```python
from build123d import *

# Parameters (mm, degrees)
ESQUISSE2_W        = 11.89
ESQUISSE2_H        = 4.55
BOSS_EXTRU_1_DEPTH = 1.5
ESQUISSE7_W        = 7.59
ESQUISSE7_H        = 3.5
BOSS_EXTRU_2_DEPTH = 1
ESQUISSE8_W        = 0.56222282
ESQUISSE8_H        = 1.99
BOSS_EXTRU_4_DEPTH = 7.3
CONG_6_R           = 0.995
ESQUISSE12_R       = 0.44
BOSS_EXTRU_5_DEPTH = 1.21


with BuildPart() as part:
    # Esquisse2 → Boss.-Extru.1 (new body)
    with BuildSketch(Plane(origin=(0, 0, 0), x_dir=(0, 0, -1), z_dir=(1, 0, 0))):
        with Locations((-5.945, 2.275)):
            Rectangle(ESQUISSE2_W, ESQUISSE2_H)
    extrude(amount=BOSS_EXTRU_1_DEPTH)

    # Esquisse7 → Boss.-Extru.2 (add)
    with BuildSketch(Plane(origin=(1.5, 0, 0), x_dir=(0, 0, -1), z_dir=(1, 0, 0))):
        with Locations((-5.945, 2.275)):
            Rectangle(ESQUISSE7_W, ESQUISSE7_H)
    extrude(amount=BOSS_EXTRU_2_DEPTH)

    # Esquisse8 → Boss.-Extru.4 (add)
    with BuildSketch(Plane(origin=(5.3, 0, 0), x_dir=(0, 0, -1), z_dir=(1, 0, 0))):
        with Locations((-6.93462953, 2.275)):
            Rectangle(ESQUISSE8_W, ESQUISSE8_H)
        with Locations((-2.97611141, 2.275)):
            Rectangle(ESQUISSE8_W, ESQUISSE8_H)
        with Locations((-8.91388859, 2.275)):
            Rectangle(ESQUISSE8_W, ESQUISSE8_H)
        with Locations((-4.95537047, 2.275)):
            Rectangle(ESQUISSE8_W, ESQUISSE8_H)
    extrude(amount=-BOSS_EXTRU_4_DEPTH)

    # Congé6
    cong_6_edges = [part.edges().sort_by_distance(p)[0] for p in [
        (5.3, 1.28, 2.97611141),
        (5.3, 1.28, 4.95537047),
        (5.3, 1.28, 6.93462953),
        (5.3, 1.28, 8.91388859),
        (5.3, 3.27, 8.91388859),
        (5.3, 3.27, 6.93462953),
        (5.3, 3.27, 4.95537047),
        (5.3, 3.27, 2.97611141),
    ]]
    fillet(cong_6_edges, radius=CONG_6_R - 0.0001)  # a hair under: the kernel refuses the full size

    # Esquisse12 → Boss.-Extru.5 (add)
    with BuildSketch(Plane.ZY):
        with Locations(Location((2.135, 4.06, 0), (0, 0, 180))):
            Circle(ESQUISSE12_R)
        with Locations(Location((9.755, 0.49, 0), (0, 0, 180))):
            Circle(ESQUISSE12_R)
    extrude(amount=BOSS_EXTRU_5_DEPTH)


solid = part.part
```
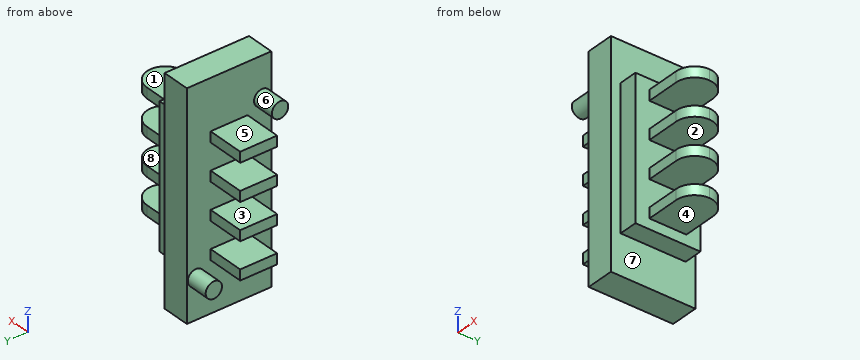
Design review of the part built by this model. Coordinates are the model's own, in mm. Face numbers are marked on the shaded views. A direction names the side the tool comes from. Give positions to 0.01 mm unless a question says otherwise; leave off trailing zeros. Order: outer loops, then holes, each group sorted by start corner. A loop starts at its lowest first (then second) coordinate and runs counter-clockwise, first axis right, second up. Notation, with made-up numbers: (5, 67.25) - (9, 67.25) arc R30 ccw to (9, 93.25) - close; hole circle Ø4 at (-34, 50). An arc over 180 degrees is marked (long way). Use a Markdown table: item, result. Add a question column.
(1) Add section C-C on x = -0.75. Give the boundary of the cut face in (y, z) (3 decimals), then the cut area to 3 significant figures.
(2) Machinability: for the marked faces 1, 2, 3 and 4, which of the approach directions +Z, -Z, +X, -X, +Y, -Y give a long, thin tool a straight path to every point of the face, cutting with its end or side? Answer none if there is none.
(3) Mouldability with a two-part tool opening along Z and no side actions: class the marked faces 5, 6, 7 and 8 as +Z half, -Z half, draft (parallel to the pull), parting line (faces both ways), or undercut.
(4) Clearance check with flat-ended pins moving along their axes: P1, Ø1, axis at x = 4.5, y = 2.5, coming from the -Z side (3 decimals); P2, Ø0.8, axis at x = 2, z = 4, coming from the +Y side (3 decimals); P3, Ø0.6, axis at x = -1, z = 9, coming from the +Y side. State where each tip first meets the part, or that it passes through.
(5) Add section A-A on x = 3. Give the boundary of the cut face in (y, z) (3 decimals).
(6) Wall thickness on probe 1 along Z at (x, y) = (3, 1.4) (3 decimals); probe 2 along X at (y, z) = (1.25, 3.5); probe 3 along Y at (x, z) = (2, 4) (3 decimals): over which ranges is each line inside the solid? List them lowest first. Write a range as [from, to].
(7) Add section B-B on y = 3.4. Give the boundary of the cut face in (x, z), then the cut area to 3 significant figures.
Report:
| question | item | result |
|---|---|---|
| 1 | outline | circle Ø0.88 at (0.49, 9.755); (1.28, 2.695) - (3.27, 2.695) - (3.27, 3.257) - (1.28, 3.257) - close; (1.28, 4.674) - (3.27, 4.674) - (3.27, 5.236) - (1.28, 5.236) - close; (1.28, 6.654) - (3.27, 6.654) - (3.27, 7.216) - (1.28, 7.216) - close; (1.28, 8.633) - (3.27, 8.633) - (3.27, 9.195) - (1.28, 9.195) - close; circle Ø0.88 at (4.06, 2.135) |
| 1 | area | 5.69 mm² |
| 2 | face 1 | +Z, +X, +Y, -Y |
| 2 | face 2 | +X, +Y, -Y |
| 2 | face 3 | -X, +Y, -Y |
| 2 | face 4 | -Z, +X, +Y, -Y |
| 3 | face 5 | +Z half |
| 3 | face 6 | parting line |
| 3 | face 7 | draft |
| 3 | face 8 | undercut |
| 4 | P1 | stops at z = 2.695 |
| 4 | P2 | stops at y = 4.025 |
| 4 | P3 | stops at y = 3.27 |
| 5 | outline | (1.28, 2.695) - (3.27, 2.695) - (3.27, 3.257) - (1.28, 3.257) - close; (1.28, 4.674) - (3.27, 4.674) - (3.27, 5.236) - (1.28, 5.236) - close; (1.28, 6.654) - (3.27, 6.654) - (3.27, 7.216) - (1.28, 7.216) - close; (1.28, 8.633) - (3.27, 8.633) - (3.27, 9.195) - (1.28, 9.195) - close |
| 6 | probe 1 | z = [2.695, 3.257], [4.674, 5.236], [6.654, 7.216], [8.633, 9.195] |
| 6 | probe 2 | x = [0, 2.5] |
| 6 | probe 3 | y = [0.525, 4.025] |
| 7 | outline | (0, 0) - (1.5, 0) - (1.5, 2.15) - (2.5, 2.15) - (2.5, 9.74) - (1.5, 9.74) - (1.5, 11.89) - (0, 11.89) - close |
| 7 | area | 25.4 mm² |
